Work out the finished part from the listing and answer in its coordinate system (mm). A direction names the side the tool comes from. Coordinates: 2 decimals unless noted, no trailing zeros. Loops run counter-clockwise (first coordinate to the right, second up) from the corner with the lowest first, then second, coordinate; pieces in that order, holes last. Notation, with made-up numbers: (39, -1) - (48, -1) arc R13 cw to (48, 3) - close; hole circle Ø10 at (79.5, 38). An arc over 180 degrees is marked (long way). Write each question's results on one line, items separated by ' | '. Start each with the question number.
1. Find the intervals of material crossed by line 1 along Z through (x, y) = (-10, -1.8); line 2 along X through (y, z) = (-1.8, 25); line 3 along X through (y, z) = (7.5, 46.5), in increasing order. Write a range as [from, to].
2. A cutting plane is placed at A-A on x = 10. Determine the outline of the cut face in (y, z).
3. Which of the six approach directions +Z, -Z, +X, -X, +Y, -Y give full straight-line access (tool end or side, diameter ignored) to faces 4 (the flat face through (3, -1.706, 25)), 5 (the cylindrical face through (8.4, -2, 26.2))?
4. A cutting plane is placed at B-B on y = -0.5. Determine the outline of the cut face in (x, z).
5. A cutting plane is placed at C-C on z = 45. Determine the outline of the cut face in (x, y), then the cut area to 3 significant figures.
6. A cutting plane is placed at D-D on z = 20. Determine the outline of the cut face in (x, y), then the cut area to 3 significant figures.
7. Each of these flat-tipped pins is pushed along its axis until it touches: P1, Ø2, axis at x = -5.5, z = 21.5, coming from the +Y side; P2, Ø2.5, axis at x = 0, z = 35, coming from the -Y side. Where does it stop, or does it pass through?
8. Determine the mould class of faces 1 (the cylindrical face through (14.75, 1.58, 6.59)), 2 (the cylindrical face through (0, -2, 37)), 3 (the cylindrical face through (-14.746, 7.493, 0.285)) for opening direction Y: released by +Y, released by -Y, zero draft, split by the parting line, or undercut.
Autodesk Inventor part; units mm, degrees
ref_plane "YZ Plane" through (0, 0, 0) normal (1, 0, 0) x (0, 1, 0)
ref_plane "XZ Plane" through (0, 0, 0) normal (0, 1, 0) x (-1, 0, 0)
ref_plane "XY Plane" through (0, 0, 0) normal (0, 0, 1) x (1, 0, 0)
sketch "Náčrt1" plane through (0, 0, 0) normal (0, 0, 1) x (1, 0, 0)
  line L0 (-14.5, 7.7937) -> (-14.5, -1.7063)
  line L1 (-14.5, -1.7063) -> (14.5, -1.7063)
  line L2 (14.5, -1.7063) -> (14.5, 7.7937)
  line L3 (14.5, 7.7937) -> (15, 7.7937)
  line L4 (15, 7.7937) -> (15, -2.2063)
  line L5 (15, -2.2063) -> (-15, -2.2063)
  line L6 (-15, -2.2063) -> (-15, 7.7937)
  line L7 (-15, 7.7937) -> (-14.5, 7.7937)
  point P0 (0, 0)
  point P1 (14.5, 3.0437)
  point P2 (-14.75, 7.7937)
  point P3 (14.75, 7.7937)
  dimension "d0" = 15
  dimension "d1" = 15
  dimension "d2" = 0.5
  dimension "d3" = 0.5
  dimension "d4" = 0.5
  dimension "d5" = 10
  dimension "d6" = 10
extrude "Vysunutí1" add sketch "Náčrt1" along normal blind 50
sketch "Náčrt2" plane through (15, -2.2063, 0) normal (1, 0, 0) x (0, 0, -1)
  circle A0 centre (-5, 5) radius 2
  line L0 (0, 0) -> (0, 10)
  point P0 (0, 2.2063)
  point P1 (0, 5)
  dimension "d9" = 4
  dimension "d10" = 5
extrude "Vysunutí2" cut sketch "Náčrt2" against normal through all
pattern_linear "Obdélníkové pole1" count 10 spacing 10 along (0, 0, 1) of "Vysunutí2"
sketch "Náčrt3" plane through (-14.5, -1.7063, 0) normal (0, 1, 0) x (1, 0, 0)
  circle A0 centre (4.5, -45) radius 2
  line L0 (29, -50) -> (0, -50)
  line L1 (-0.5, 0) -> (-0.5, -50)
  point P0 (14.5, 0)
  dimension "d16" = 4
  dimension "d17" = 5
  dimension "d18" = 5
extrude "Vysunutí3" cut sketch "Náčrt3" against normal through all
pattern_linear "Obdélníkové pole2" count 10 spacing 10 along (0, 0, -1) count 5 spacing 10 along (1, 0, 0) of "Vysunutí3"
fillet "Zaoblení1" radius 1 1 edges at (-14.75, 7.7937, 50)
fillet "Zaoblení2" radius 1 1 edges at (14.75, 7.7937, 50)
fillet "Zaoblení3" radius 1 2 edges at (14.75, 7.7937, 0) (-14.75, 7.7937, 0)
properties part number "1024 modra"
Values:
1) line 1: [0, 3], [7, 13], [17, 23], [27, 33], [37, 43], [47, 50] | line 2: [-15, -12], [-8, -2], [2, 8], [12, 15] | line 3: [-15, -14.5], [14.5, 15]
2) outline: (-2.21, 0) - (-1.71, 0) - (-1.71, 3) - (-2.21, 3) - close; (-2.21, 7) - (-1.71, 7) - (-1.71, 13) - (-2.21, 13) - close; (-2.21, 17) - (-1.71, 17) - (-1.71, 23) - (-2.21, 23) - close; (-2.21, 27) - (-1.71, 27) - (-1.71, 33) - (-2.21, 33) - close; (-2.21, 37) - (-1.71, 37) - (-1.71, 43) - (-2.21, 43) - close; (-2.21, 47) - (-1.71, 47) - (-1.71, 50) - (-2.21, 50) - close
3) face 4: +Z, -Z, +Y | face 5: +Y, -Y
4) outline: (-15, 0) - (-14.5, 0) - (-14.5, 50) - (-15, 50) - close; (14.5, 0) - (15, 0) - (15, 50) - (14.5, 50) - close
5) outline: (-15, -2.21) - (-12, -2.21) - (-12, -1.71) - (-14.5, -1.71) - (-14.5, 0.79) - (-15, 0.79) - close; (-15, 4.79) - (-14.5, 4.79) - (-14.5, 7.79) - (-15, 7.79) - close; (-8, -2.21) - (-2, -2.21) - (-2, -1.71) - (-8, -1.71) - close; (2, -2.21) - (8, -2.21) - (8, -1.71) - (2, -1.71) - close; (12, -2.21) - (15, -2.21) - (15, 0.79) - (14.5, 0.79) - (14.5, -1.71) - (12, -1.71) - close; (14.5, 4.79) - (15, 4.79) - (15, 7.79) - (14.5, 7.79) - close | area: 14.5 mm^2
6) outline: (-15, -2.21) - (15, -2.21) - (15, 7.79) - (14.5, 7.79) - (14.5, -1.71) - (-14.5, -1.71) - (-14.5, 7.79) - (-15, 7.79) - close | area: 24.5 mm^2
7) P1: y = -1.71 | P2: through
8) face 1: undercut | face 2: zero draft | face 3: released by +Y
